Could you check a few things on this model? Use its own coordinates, in mm. A direction names the side the tool comes from. Give positions to 0.01 mm unless a question says otherwise; leave off trailing zeros. Write each loop counter-clockwise with the first axis right and the second up, starting at its lowest first coordinate (ties: lowest second). Pieces come first, ordered by that corner, then holes. Notation, with made-up numbers: (15.5, -3.5) - (70.5, -3.5) arc R15 ccw to (70.5, 10.5) - close; hole circle Ø10 at (-8, -6). An arc over 180 degrees is marked (long way). Answer as a JSON object with one key per item and string values. Group by question number.
```python
from build123d import *

# Parameters (mm, degrees)
F1_DEPTH       = 35
F2_DEPTH       = 5
F3_W           = 33.611692
F3_H           = 49.436976
F4_DEPTH       = 25
F5_W           = 28.51793
F5_H           = 14.842174
F6_DEPTH       = 10
F9_D           = 5
F9_CSINK_D     = 12.1
F9_CSINK_ANGLE = 90
F10_W          = 36.775354
F10_H          = 36.023068
F11_DEPTH      = 25


with BuildPart() as f1:
    # F0 (on Top) → F1 (new body)
    with BuildSketch(Plane.XY):
        Polygon((-20, 30), (20, 30), (30, 30), (30, 40), (-30, 40), (-30, -40), (30, -40), (30, -30), (20, -30), (-20, -30), align=None)
    extrude(amount=F1_DEPTH)

    # F0 (on Top) → F2 (join)
    with BuildSketch(Plane.XY):
        Polygon((30, 30), (20, 30), (-20, 30), (-20, -30), (20, -30), (30, -30), align=None)
    extrude(amount=F2_DEPTH)

    # F3 (on face) → F4 (cut)
    with BuildSketch(Plane.XY.offset(5)):
        Rectangle(F3_W, F3_H)
    extrude(amount=-F4_DEPTH, mode=Mode.SUBTRACT)

    # F5 (on face) → F6 (join)
    with BuildSketch(Plane.XY.offset(35)):
        with Locations((0, -47.421087)):
            Rectangle(F5_W, F5_H)
        with Locations((0, 47.421087)):
            Rectangle(F5_W, F5_H)
    extrude(amount=-F6_DEPTH)

    # F9 (through all)
    with Locations(Plane(origin=(0, 0, 25), x_dir=(1, 0, 0), z_dir=(0, 0, -1))):
        with Locations((7.129482, 47.421087), (-7.129482, 47.421087), (-7.129482, -47.421087), (7.129482, -47.421087)):
            CounterSinkHole(F9_D / 2, F9_CSINK_D / 2, counter_sink_angle=F9_CSINK_ANGLE)

    # F10 (on face) → F11 (cut)
    with BuildSketch(Plane(origin=(-30, 0, 0), x_dir=(0, -1, 0), z_dir=(-1, 0, 0))):
        with Locations((0, 35)):
            Rectangle(F10_W, F10_H)
    extrude(amount=-F11_DEPTH, mode=Mode.SUBTRACT)


solid = f1.part
```
(1) I want a section at A-A, the plane y = 20. Please give me the cut outline in (x, z).
(2) I want a section at C-C, the plane x = -23.5. Please give me the cut outline in (y, z).
(3) I need wall thicknesses on L1, parallel to Y at x = 3.5, z = 12; L2, parallel to Y at x = 2.5, z = 31; L3, parallel to X at y = -20, z = 3. Which ranges of each line are inside material? Lowest first, please.
(4) If we mould it in two halves opening along X, with no side actions, what happens to faces 4 (the flat face through (-20, 1, 0)), 5 (the flat face through (0, -24.718, 3)), 6 (the flat face through (-30, 1, 13)), 7 (the flat face through (14.259, -48, 30))? For each: +X half, -X half, draft (parallel to the pull), parting line (faces both ways), or undercut.
(5) I want a section at B-B, the plane z = 21. Please give me the cut outline in (x, y), and give its area (3 significant figures).
(6) Will these pins go through, and if not, where does the flat tip stop? P1, Ø6, axis at x = -22, z = 23.5, coming from the -Y side; P2, Ø1.5, axis at y = 22.5, z = 18.5, coming from the +X side; P3, Ø3, axis at x = -7.13, y = 47.42, coming from the +Z side; P4, Ø1.5, axis at x = 10.5, z = 18.5, coming from the +Y side.
(7) I want a section at D-D, the plane z = 31. Please give me the cut outline in (x, y).
(8) For faces 1 (the flat face through (-14.259, -48, 30)), 2 (the flat face through (5, 30, 20)), 3 (the flat face through (-25, -18.388, 26)), which set-ups out of +Z, -Z, +X, -X, +Y, -Y let a thin tool reach every point of the face, with its end or its side?
Entries:
{
 "1": {"outline": "(-30, 0) - (-16.81, 0) - (-16.81, 5) - (-20, 5) - (-20, 35) - (-30, 35) - close; (16.81, 0) - (30, 0) - (30, 5) - (16.81, 5) - close"},
 "2": {"outline": "(-40, 0) - (40, 0) - (40, 35) - (18.39, 35) - (18.39, 16.99) - (-18.39, 16.99) - (-18.39, 35) - (-40, 35) - close"},
 "3": {"L1": "-40 to -30, 30 to 40", "L2": "-54.84 to -30, 30 to 54.84", "L3": "-30 to -16.81, 16.81 to 30"},
 "4": {"face 4": "draft", "face 5": "undercut", "face 6": "-X half", "face 7": "+X half"},
 "5": {"outline": "(-30, -40) - (30, -40) - (30, -30) - (-20, -30) - (-20, -18.39) - (-30, -18.39) - close; (-30, 18.39) - (-20, 18.39) - (-20, 30) - (30, 30) - (30, 40) - (-30, 40) - close", "area": "1,430 mm^2"},
 "6": {"P1": "y = -40", "P2": "x = -20", "P3": "through", "P4": "y = 40"},
 "7": {"outline": "(-30, -40) - (-14.26, -40) - (-14.26, -54.84) - (14.26, -54.84) - (14.26, -40) - (30, -40) - (30, -30) - (-20, -30) - (-20, -18.39) - (-30, -18.39) - close; (-30, 18.39) - (-20, 18.39) - (-20, 30) - (30, 30) - (30, 40) - (14.26, 40) - (14.26, 54.84) - (-14.26, 54.84) - (-14.26, 40) - (-30, 40) - close; hole circle Ø5 at (-7.13, -47.42); hole circle Ø5 at (-7.13, 47.42); hole circle Ø5 at (7.13, -47.42); hole circle Ø5 at (7.13, 47.42)"},
 "8": {"face 1": "+Z, -Z, -X, -Y", "face 2": "+Z, +X", "face 3": "+Z, +X, -X"}
}
